```python
from build123d import *

# Parameters (mm, degrees)
SKETCH1_W           = 93.98
SKETCH1_H           = 63.5
BOSS_EXTRUDE1_DEPTH = 30.48
FILLET1_R           = 5.08
BOSS_EXTRUDE2_START = -12.7
BOSS_EXTRUDE2_DEPTH = 50.8
SKETCH4_W           = 63.5
SKETCH4_H           = 16.51
BOSS_EXTRUDE3_DEPTH = 1.778
SKETCH5_W           = 58.42
SKETCH5_H           = 8.89
BOSS_EXTRUDE4_DEPTH = 12.7


with BuildPart() as part:
    # Sketch1 → Boss-Extrude1 (new body)
    with BuildSketch(Plane(origin=(0, 0, 0), x_dir=(1, 0, 0), z_dir=(0, 1, 0))):
        Rectangle(SKETCH1_W, SKETCH1_H)
    extrude(amount=BOSS_EXTRUDE1_DEPTH)

    # Fillet1
    fillet1_edges = [part.edges().sort_by_distance(p)[0] for p in [
        (46.99, 15.24, 31.75),
        (-46.99, 15.24, 31.75),
        (-46.99, 15.24, -31.75),
        (46.99, 15.24, -31.75),
    ]]
    fillet(fillet1_edges, radius=FILLET1_R)

    # Sketch2 → Boss-Extrude2 (add)
    with BuildSketch(Plane(origin=(46.99, 0, 0), x_dir=(0, 0, -1), z_dir=(1, 0, 0)).offset(BOSS_EXTRUDE2_START)):
        with BuildLine():
            Line((-38.1, 31.75), (-38.1, 69.85))
            ThreePointArc((-38.1, 69.85), (-57.15, 88.9), (-76.2, 69.85))
            Line((-76.2, 69.85), (-76.2, 0))
            Line((-76.2, 0), (-77.47, 0))
            Line((-77.47, 0), (-77.47, 69.85))
            ThreePointArc((-77.47, 69.85), (-57.15, 90.17), (-36.83, 69.85))
            Line((-36.83, 69.85), (-36.83, 31.75))
            ThreePointArc((-36.83, 31.75), (-35.342102448, 28.157897552), (-31.75, 26.67))
            Line((-31.75, 26.67), (-31.75, 25.4))
            ThreePointArc((-31.75, 25.4), (-36.240128061, 27.259871939), (-38.1, 31.75))
        make_face()
    extrude(amount=-BOSS_EXTRUDE2_DEPTH)

    # Sketch4 → Boss-Extrude3 (add)
    with BuildSketch(Plane.XZ):
        with Locations((8.89, 76.835)):
            Rectangle(SKETCH4_W, SKETCH4_H)
    extrude(amount=BOSS_EXTRUDE3_DEPTH)

    # Sketch5 → Boss-Extrude4 (add)
    with BuildSketch(Plane(origin=(0, 0, 0), x_dir=(1, 0, 0), z_dir=(0, 1, 0))):
        with Locations((8.89, -76.835)):
            Rectangle(SKETCH5_W, SKETCH5_H)
    extrude(amount=BOSS_EXTRUDE4_DEPTH)


solid = part.part
```
Input: part model. Units: mm. Frame: model coordinates. A direction names the side the tool comes from. Give positions to 0.01 mm unless a question says otherwise; leave off trailing zeros. Order: outer loops, then holes, each group sorted by start corner. A loop starts at its lowest first (then second) coordinate and runs counter-clockwise, first axis right, second up. Notation, with made-up numbers: (-38, 23) - (6, 23) arc R23 ccw to (6, 41) - close; hole circle Ø9 at (35.5, -33). An arc over 180 degrees is marked (long way). One line per item, written item: value.
1. Line query: probe 1 along Z at (x, y) = (30, 43.5); probe 2 along Y at (x, z) = (6, -20.5); probe 3 along Y at (x, z) = (-10, 73). Output: solid intervals per line, ascending.
Determined:
probe 1: 36.83 to 38.1, 76.2 to 77.47
probe 2: 0 to 30.48
probe 3: -1.78 to 12.7, 80.42 to 82.57
2. Cut plane D-D, the plane y = 51. Output: boundary loops of the cut face in (x, z), and give its area (3 significant figures).
Determined:
outline: (-16.51, 36.83) - (34.29, 36.83) - (34.29, 38.1) - (-16.51, 38.1) - close; (-16.51, 76.2) - (34.29, 76.2) - (34.29, 77.47) - (-16.51, 77.47) - close
area: 129 mm2
3. Cut plane C-C, the plane z = 74. Output: boundary loops of the cut face in (x, y), and give its area (3 significant figures).
Determined:
outline: (-22.86, -1.78) - (40.64, -1.78) - (40.64, 0) - (38.1, 0) - (38.1, 12.7) - (-20.32, 12.7) - (-20.32, 0) - (-22.86, 0) - close; (-16.51, 78.74) - (34.29, 78.74) - (34.29, 81.21) - (-16.51, 81.21) - close
area: 980 mm2
4. Cut plane B-B, the plane x = 7.5. Output: boundary loops of the cut face in (y, z).
Determined:
outline: (-1.78, 68.58) - (0, 68.58) - (0, 72.39) - (12.7, 72.39) - (12.7, 76.2) - (69.85, 76.2) arc R19.05 cw to (69.85, 38.1) - (31.75, 38.1) arc R6.35 ccw to (25.4, 31.75) - (0, 31.75) - (0, -31.75) - (30.48, -31.75) - (30.48, 31.75) - (26.67, 31.75) arc R5.08 cw to (31.75, 36.83) - (69.85, 36.83) arc R20.32 ccw to (69.85, 77.47) - (12.7, 77.47) - (12.7, 81.28) - (0, 81.28) - (0, 85.09) - (-1.78, 85.09) - close
5. Pin query (flat end, axial travel): pin 1 Ø7 at (x, z) = (1.5, 75) entering from +Y; pin 2 Ø6.5 at (x, y) = (-5.5, 7.5) entering from +Z; pin 3 Ø2 at (y, z) = (-1, 78.5) entering from -X; pin 4 Ø6 at (x, y) = (-22.5, 33) entering from -Z. Return the tip coordinate at first contact, or that it passes through.
Determined:
pin 1: y = 84.24
pin 2: z = 81.28
pin 3: x = -22.86
pin 4: z = -31.75
6. Draft query along Z for faces 1 (the face through (8, -1.778, 77)), 2 (the face through (9, 41, 77.47)), 3 (the face through (-1, 15, 31.75)), 4 (the face through (9.246, 28.198, 35.381)). Return one class per face: released by +Z, released by -Z, zero draft, split by the parting line, or undercut.
Determined:
face 1: zero draft
face 2: released by +Z
face 3: undercut
face 4: undercut
7. Cut plane A-A, the plane y = 7. Output: boundary loops of the cut face in (x, z), and give its area (3 significant figures).
Determined:
outline: (-46.99, -26.67) arc R5.08 ccw to (-41.91, -31.75) - (41.91, -31.75) arc R5.08 ccw to (46.99, -26.67) - (46.99, 26.67) arc R5.08 ccw to (41.91, 31.75) - (-41.91, 31.75) arc R5.08 ccw to (-46.99, 26.67) - close; (-20.32, 72.39) - (38.1, 72.39) - (38.1, 81.28) - (-20.32, 81.28) - close
area: 6,460 mm2
8. Reachability of faces 5 (the face through (-16.51, 57, 77)), 6 (the face through (-1, 30.48, 0)), 7 (the face through (-1, 0, 0)), 8 (the face through (8, 6, 72.39)), 9 (the face through (34.29, 57, 77)) from +Z, -Z, +X, -X, +Y, -Y: full face, straight path, thin tool, end or side. Return the list, or none.
Determined:
face 5: +Z, -X, +Y
face 6: -Z, +X, -X, +Y
face 7: -Z, +X, -X, -Y
face 8: +X, -X
face 9: +Z, +X, +Y
